The listing builds one solid part. Answer for the finished solid, in the listing's coordinates (mm). A direction names the side the tool comes from. Give positions to 0.01 mm unless a question says otherwise; leave off trailing zeros. Loops run counter-clockwise (first coordinate to the right, second up) from the corner with the lowest first, then second, coordinate; pieces in that order, holes last. Notation, with made-up numbers: M 28,49.25 L 53,49.25 A20 cw 53,62.25 Z; hole C 7.25,48.25 d8. An arc over 180 degrees is marked long. One line per item, written item: value. Start each with the question number.
Q1. For faces 1 (the flat face through (35, 0, 18)), 2 (the flat face through (-1, 0, 0)), determine the directions among +Z, -Z, +X, -X, +Y, -Y from which every point of the face is accessible in a straight line to the end or side of a thin tool.
Q2. A cutting plane is placed at B-B, the plane x = -7.5. Determine the outline of the cut face in (y, z), and give its area (3 significant figures).
Q3. A flat-ended cylindrical pin translates along its axis: pin 1 (25 mm diameter, centred on x = -6, y = -7.5, fed in from +Z). Find the tip coordinate at first contact, or state that the pin passes through.
Q4. The mould has two halves that part along X. Classify faces 3 (the flat face through (0, 26.5, 17)), 4 (the flat face through (-35, 0, 18)), 5 (the cylindrical face through (-35.07, -25, 17.26)): +X half, -X half, draft (parallel to the pull), parting line (faces both ways), or undercut.
Q5. A cutting plane is placed at C-C, the plane y = 2.5. Determine the outline of the cut face in (x, z).
Q6. A cutting plane is placed at A-A, the plane z = 33. Determine the outline of the cut face in (x, y).
Q7. Consider L1, parallel to X at y = -18, z = 30.5; L2, parallel to Y at x = -7.5, z = 26.5; L3, parallel to Z at x = 28, y = 4. Determine where each line is inside the solid, lowest interval first.
from build123d import *

# Parameters (mm, degrees)
F1_DEPTH = 2
F2_DEPTH = 35


with BuildPart() as f1:
    # F0 (on Top) → F1 (new body)
    with BuildSketch(Plane.XY):
        with BuildLine():
            Line((31.5, 26.5), (-31.5, 26.5))
            ThreePointArc((-31.5, 26.5), (-35.0355339059, 25.0355339059), (-36.5, 21.5))
            Line((-36.5, 21.5), (-36.5, -21.5))
            ThreePointArc((-36.5, -21.5), (-35.0355339059, -25.0355339059), (-31.5, -26.5))
            Line((-31.5, -26.5), (31.5, -26.5))
            ThreePointArc((31.5, -26.5), (35.0355339059, -25.0355339059), (36.5, -21.5))
            Line((36.5, -21.5), (36.5, 21.5))
            ThreePointArc((36.5, 21.5), (35.0355339059, 25.0355339059), (31.5, 26.5))
        make_face()
        with BuildLine():
            ThreePointArc((-35, 20), (-33.5355339059, 23.5355339059), (-30, 25))
            Line((-30, 25), (30, 25))
            ThreePointArc((30, 25), (33.5355339059, 23.5355339059), (35, 20))
            Line((35, 20), (35, -20))
            ThreePointArc((35, -20), (33.5355339059, -23.5355339059), (30, -25))
            Line((30, -25), (-30, -25))
            ThreePointArc((-30, -25), (-33.5355339059, -23.5355339059), (-35, -20))
            Line((-35, -20), (-35, 20))
        make_face(mode=Mode.SUBTRACT)
        with BuildLine():
            Line((30, 25), (-30, 25))
            ThreePointArc((-30, 25), (-33.5355339059, 23.5355339059), (-35, 20))
            Line((-35, 20), (-35, -20))
            ThreePointArc((-35, -20), (-33.5355339059, -23.5355339059), (-30, -25))
            Line((-30, -25), (30, -25))
            ThreePointArc((30, -25), (33.5355339059, -23.5355339059), (35, -20))
            Line((35, -20), (35, 20))
            ThreePointArc((35, 20), (33.5355339059, 23.5355339059), (30, 25))
        make_face()
    extrude(amount=F1_DEPTH)

    # F0 (on Top) → F2 (join)
    with BuildSketch(Plane.XY):
        with BuildLine():
            Line((31.5, 26.5), (-31.5, 26.5))
            ThreePointArc((-31.5, 26.5), (-35.0355339059, 25.0355339059), (-36.5, 21.5))
            Line((-36.5, 21.5), (-36.5, -21.5))
            ThreePointArc((-36.5, -21.5), (-35.0355339059, -25.0355339059), (-31.5, -26.5))
            Line((-31.5, -26.5), (31.5, -26.5))
            ThreePointArc((31.5, -26.5), (35.0355339059, -25.0355339059), (36.5, -21.5))
            Line((36.5, -21.5), (36.5, 21.5))
            ThreePointArc((36.5, 21.5), (35.0355339059, 25.0355339059), (31.5, 26.5))
        make_face()
        with BuildLine():
            ThreePointArc((-35, 20), (-33.5355339059, 23.5355339059), (-30, 25))
            Line((-30, 25), (30, 25))
            ThreePointArc((30, 25), (33.5355339059, 23.5355339059), (35, 20))
            Line((35, 20), (35, -20))
            ThreePointArc((35, -20), (33.5355339059, -23.5355339059), (30, -25))
            Line((30, -25), (-30, -25))
            ThreePointArc((-30, -25), (-33.5355339059, -23.5355339059), (-35, -20))
            Line((-35, -20), (-35, 20))
        make_face(mode=Mode.SUBTRACT)
    extrude(amount=F2_DEPTH)


solid = f1.part
Answer block:
1. face 1: +Z
1. face 2: -Z, +X, -X, +Y, -Y
2. outline: M -26.5,0 L 26.5,0 L 26.5,35 L 25,35 L 25,2 L -25,2 L -25,35 L -26.5,35 Z
2. area: 205 mm^2
3. pin 1: z = 2
4. face 3: draft
4. face 4: undercut
4. face 5: -X half
5. outline: M -36.5,0 L 36.5,0 L 36.5,35 L 35,35 L 35,2 L -35,2 L -35,35 L -36.5,35 Z
6. outline: M -36.5,-21.5 A5 ccw -31.5,-26.5 L 31.5,-26.5 A5 ccw 36.5,-21.5 L 36.5,21.5 A5 ccw 31.5,26.5 L -31.5,26.5 A5 ccw -36.5,21.5 Z; hole M -35,-20 A5 ccw -30,-25 L 30,-25 A5 ccw 35,-20 L 35,20 A5 ccw 30,25 L -30,25 A5 ccw -35,20 Z
7. L1: -36.5 to -35, 35 to 36.5
7. L2: -26.5 to -25, 25 to 26.5
7. L3: 0 to 2
